Verification items for the finished model (mm, model axes). A direction names the side the tool comes from. Give positions to 0.01 mm unless a question says otherwise; leave off trailing zeros. Order: outer loops, then holes, each group sorted by start corner. A loop starts at its lowest first (then second) coordinate and runs counter-clockwise, first axis right, second up. Notation, with made-up numbers: (83.25, 53.25) -> (96.25, 53.25) arc R25 ccw to (96.25, 71.25) -> close; hole circle Ø4 at (47, 57). An arc over 180 degrees is marked (long way). One line per question, with ' | ' between items. Start each with the question number.
Q1. Section check C-C on y = 5. Give the number of separate pieces and of enclosed holes in the cut face, plus the area to 3 significant figures.
Q2. Access from +Z, -Z, +X, -X, +Y, -Y to the whole of each face (thin tool, end or side, straight path). Record for faces 5 (the cylindrical face through (-7.559, 18.089, 5.796)), 6 (the flat face through (0, 43.18, 0)), 7 (the cylindrical face through (3.03, 7.3, -11.03)), 8 (the flat face through (-10, 6.35, 0)), 9 (the flat face through (0, 0, 0)).
Q3. Go/stop test with flat-tipped pins: pin 1 (12 mm diameter, centred on y = 27.5, z = -2, fed in from -X); pin 2 (1.6 mm diameter, centred on x = 9.5, z = -0.5, fed in from -Y); pin 3 (5 mm diameter, centred on x = 1.5, y = 6.5, fed in from +Z); pin 4 (12 mm diameter, centred on x = 9, y = 10, fed in from -Z). Record where each tip stops, or that it passes through.
Q4. Mould release check, pull along Z, two halves, no side actions. Record for faces 1 (the cylindrical face through (3.03, 7.3, 9.48)), 2 (the flat face through (0, 6, 6.35)), 3 (the cylindrical face through (-2.75, 30.79, 12.4)), 4 (the cylindrical face through (8.01, 3.13, -0.48)): released by +Z, released by -Z, zero draft, split by the parting line, or undercut.
Q5. Section check A-A on x = 10.5. Record the cut outline in (y, z), plus the area to 3 significant figures.
Q6. Material ranges on probe 1 along Y at (x, z) = (0, -11.4) (1 decimal); probe 2 along X at (y, z) = (2.5, 0); probe 3 along Y at (x, z) = (8.25, 8.5), recorded low to high. Write a range as [from, to].
from build123d import *

# Parameters (mm, degrees)
SKETCH1_R           = 12.7
BOSS_EXTRUDE1_DEPTH = 17.4625
SKETCH2_R           = 9.525
BOSS_EXTRUDE2_DEPTH = 1.27
SKETCH3_R           = 12.7
BOSS_EXTRUDE3_DEPTH = 24.4475
CUT_EXTRUDE1_REACH  = 21.05
CUT_EXTRUDE1_START  = 6.35
SKETCH4_R           = 3.175
CUT_EXTRUDE2_REACH  = 24.098
CUT_EXTRUDE2_START  = -9.398
SKETCH5_R           = 3.175
SKETCH6_R           = 1.5875
CUT_EXTRUDE3_DEPTH  = 6.35


with BuildPart() as part:
    # Sketch1 → Boss-Extrude1 (new body)
    with BuildSketch(Plane(origin=(0, 0, 0), x_dir=(1, 0, 0), z_dir=(0, 1, 0))):
        Circle(SKETCH1_R)
    extrude(amount=BOSS_EXTRUDE1_DEPTH)

    # Sketch2 → Boss-Extrude2 (add)
    with BuildSketch(Plane(origin=(0, 17.4625, 0), x_dir=(1, 0, 0), z_dir=(0, 1, 0))):
        Circle(SKETCH2_R)
    extrude(amount=BOSS_EXTRUDE2_DEPTH)

    # Sketch3 → Boss-Extrude3 (add)
    with BuildSketch(Plane(origin=(0, 18.7325, 0), x_dir=(1, 0, 0), z_dir=(0, 1, 0))):
        Circle(SKETCH3_R)
    extrude(amount=BOSS_EXTRUDE3_DEPTH)

    # Sketch4 → Cut-Extrude1 (cut, up to next)
    with BuildSketch(Plane.XY.offset(CUT_EXTRUDE1_START), mode=Mode.PRIVATE) as cut_extrude1_sk1:
        with Locations((0, 6.35)):
            Circle(SKETCH4_R)
    cut_extrude1_tool1 = extrude(cut_extrude1_sk1.sketch, amount=CUT_EXTRUDE1_REACH, mode=Mode.PRIVATE) & part.part
    add(cut_extrude1_tool1.solids().sort_by_distance((0, 6.35, 6.35))[0], mode=Mode.SUBTRACT)

    # Sketch5 → Cut-Extrude2 (cut, up to next)
    with BuildSketch(Plane.XY.offset(CUT_EXTRUDE2_START), mode=Mode.PRIVATE) as cut_extrude2_sk1:
        with Locations((0, 6.35)):
            Circle(SKETCH5_R)
    cut_extrude2_tool1 = extrude(cut_extrude2_sk1.sketch, amount=-CUT_EXTRUDE2_REACH, mode=Mode.PRIVATE) & part.part
    add(cut_extrude2_tool1.solids().sort_by_distance((0, 6.35, -9.398))[0], mode=Mode.SUBTRACT)

    # Sketch6 → Cut-Extrude3 (cut)
    with BuildSketch(Plane(origin=(0, 0, 0), x_dir=(-1, 0, 0), z_dir=(0, -1, 0))):
        with Locations((-9.525, 0)):
            Circle(SKETCH6_R)
        with Locations((9.525, 0)):
            Circle(SKETCH6_R)
    extrude(amount=-CUT_EXTRUDE3_DEPTH, mode=Mode.SUBTRACT)


solid = part.part
Filled in:
1) separate pieces: 1 | enclosed holes: 2 | area: 437 mm²
2) face 5: none | face 6: +Z, -Z, +X, -X, +Y | face 7: -Z | face 8: -Y | face 9: +Z, -Z, +X, -X, -Y
3) pin 1: x = -12.7 | pin 2: y = 6.35 | pin 3: z = 12.58 | pin 4: z = -12.34
4) face 1: zero draft | face 2: released by +Z | face 3: split by the parting line | face 4: undercut
5) outline: (0, -7.14) -> (17.46, -7.14) -> (17.46, 7.14) -> (0, 7.14) -> (0, 1.25) -> (6.35, 1.25) -> (6.35, -1.25) -> (0, -1.25) -> close; (18.73, -7.14) -> (43.18, -7.14) -> (43.18, 7.14) -> (18.73, 7.14) -> close | area: 583 mm²
6) probe 1: [0, 3.2], [9.5, 17.5], [18.7, 43.2] | probe 2: [-12.7, -11.11], [-7.94, 7.94], [11.11, 12.7] | probe 3: [0, 17.46], [18.73, 43.18]
